Work out the finished part from the listing and answer in its coordinate system (mm). Coordinates: 2 decimals unless noted, no trailing zeros.
1. The part is cut by section A-A, the plane z = -34.6. Count the separate pieces of the cut face and the enclosed holes in it, then the cut area to 3 significant figures.
2. Flat-ended cylindrical pins translate along their axes: pin 1 Ø1 at (x, y) = (-28.5, -25.5) entering from +Z; pin 2 Ø1.5 at (y, z) = (-20.5, -35.5) entering from +X; pin 3 Ø2 at (x, y) = (19.5, -22.5) entering from +Z. Find the tip coordinate at first contact, or state that the pin passes through.
3. Find the intervals of material crossed by probe 1 along X at (y, z) = (-22.75, -34.7); probe 2 along X at (y, z) = (-23, -36.3); probe 3 along Y at (x, z) = (-55.5, -36.2), in increasing order.
```python
from build123d import *

# Parameters (mm, degrees)
BOX126_W                          = 90
BOX126_H                          = 9
BOX126_DEPTH                      = 4
BOX125_W                          = 40
BOX125_H                          = 10
BOX125_DEPTH                      = 10
CYLINDER211_R                     = 3.25
CYLINDER211_DEPTH                 = 3.5
CYLINDER212_R                     = 0.6
CYLINDER212_DEPTH                 = 9.5
CYLINDER210_R                     = 0.6
CYLINDER210_DEPTH                 = 9.5
CYLINDER209_R                     = 3.25
CYLINDER209_DEPTH                 = 3.5
PAD016_DEPTH                      = 4
FILLET087_R                       = 3
PART_MIRRORING004_PLACEMENT_ANGLE = 180
BOX123_W                          = 40
BOX123_H                          = 10
BOX123_DEPTH                      = 10
CYLINDER205_R                     = 3.25
CYLINDER205_DEPTH                 = 3.5
CYLINDER208_R                     = 0.6
CYLINDER208_DEPTH                 = 9.5
CYLINDER206_R                     = 0.6
CYLINDER206_DEPTH                 = 9.5
CYLINDER207_R                     = 3.25
CYLINDER207_DEPTH                 = 3.5
PAD017_DEPTH                      = 4
FILLET086_R                       = 3


with BuildPart() as obj1:
    # Box126 → Box126 (new body)
    with BuildSketch(Plane(origin=(-63, -27.5, -41), x_dir=(1, 0, 0), z_dir=(0, 0, 1))):
        with Locations((45, 4.5)):
            Rectangle(BOX126_W, BOX126_H)
    extrude(amount=BOX126_DEPTH)


with BuildPart() as obj2:
    # Box125 → Box125 (new body)
    with BuildSketch(Plane(origin=(-14, -72, -42), x_dir=(1, 0, 0), z_dir=(0, 0, 1))):
        with Locations((20, 5)):
            Rectangle(BOX125_W, BOX125_H)
    extrude(amount=BOX125_DEPTH)


with BuildPart() as zylinder211:
    # Cylinder211 → Cylinder211 (new body)
    with BuildSketch(Plane(origin=(-52.5, 23, -36), x_dir=(1, 0, 0), z_dir=(0, 0, 1))):
        Circle(CYLINDER211_R)
    extrude(amount=CYLINDER211_DEPTH)


with BuildPart() as zylinder212:
    # Cylinder212 → Cylinder212 (new body)
    with BuildSketch(Plane(origin=(16.5, 23, -39), x_dir=(1, 0, 0), z_dir=(0, 0, 1))):
        Circle(CYLINDER212_R)
    extrude(amount=CYLINDER212_DEPTH)


with BuildPart() as zylinder210:
    # Cylinder210 → Cylinder210 (new body)
    with BuildSketch(Plane(origin=(-52.5, 23, -39), x_dir=(1, 0, 0), z_dir=(0, 0, 1))):
        Circle(CYLINDER210_R)
    extrude(amount=CYLINDER210_DEPTH)


with BuildPart() as fusion135:
    # Cylinder209 → Cylinder209 (new body)
    with BuildSketch(Plane(origin=(16.5, 23, -36), x_dir=(1, 0, 0), z_dir=(0, 0, 1))):
        Circle(CYLINDER209_R)
    extrude(amount=CYLINDER209_DEPTH)

    # Fusion135: union Zylinder211, Zylinder212, Zylinder210
    add(zylinder211.part)
    add(zylinder212.part)
    add(zylinder210.part)


with BuildPart() as cut090:
    # Sketch017 → Pad016 (new body)
    with BuildSketch(Plane.XY):
        with BuildLine():
            add(Edge.make_bspline(
                [(-48.5, 19), (-18, 24), (12.5, 19)],
                knots=[0, 0, 0, 1, 1, 1], degree=2))
            Line((-48.5, 19), (-57, 19))
            Line((-57, 19), (-57, 27))
            Line((-57, 27), (-48.5, 27))
            add(Edge.make_bspline(
                [(-48.5, 27), (-18, 22), (12.5, 27)],
                knots=[0, 0, 0, 1, 1, 1], degree=2))
            Line((12.5, 27), (21, 27))
            Line((21, 27), (21, 19))
            Line((21, 19), (12.5, 19))
        make_face()
    extrude(amount=PAD016_DEPTH)


with BuildPart() as cut090_1:
    # Body007 placement: moved
    add(cut090.part.moved(Location((0, 0, -38))))

    # Cut088: cut Fusion135
    add(fusion135.part, mode=Mode.SUBTRACT)

    # Fillet087
    fillet087_edges = [cut090_1.edges().sort_by_distance(p)[0] for p in [
        (-57, 19, -36),
        (21, 19, -36),
        (-57, 27, -36),
        (21, 27, -36),
    ]]
    fillet(fillet087_edges, radius=FILLET087_R)


with BuildPart() as cut090_2:
    # Fillet087 placement: moved
    add(cut090_1.part.moved(Location((0, -90, 0))))

    # Cut090: cut obj2
    add(obj2.part, mode=Mode.SUBTRACT)


with BuildPart() as cut090_3:
    # Cut090 placement: moved
    add(cut090_2.part.moved(Location((-5, 35, 0))))


with BuildPart() as part_mirroring004:
    # Part__Mirroring004: instance of Cut090
    add(cut090_3.part.mirror(Plane(origin=(-40.5, -8e-06, -36), x_dir=(1, 0, 0), z_dir=(0, 1, 0))))


with BuildPart() as part_mirroring004_1:
    # Part__Mirroring004 placement: moved
    add(part_mirroring004.part.moved(Location((-38, 9, 0))).rotate(Axis((-38, 9, 0), (0, 0, 1)), PART_MIRRORING004_PLACEMENT_ANGLE))


with BuildPart() as obj3:
    # Box123 → Box123 (new body)
    with BuildSketch(Plane(origin=(-14, -72, -42), x_dir=(1, 0, 0), z_dir=(0, 0, 1))):
        with Locations((20, 5)):
            Rectangle(BOX123_W, BOX123_H)
    extrude(amount=BOX123_DEPTH)


with BuildPart() as zylinder205:
    # Cylinder205 → Cylinder205 (new body)
    with BuildSketch(Plane(origin=(-52.5, 23, -36), x_dir=(1, 0, 0), z_dir=(0, 0, 1))):
        Circle(CYLINDER205_R)
    extrude(amount=CYLINDER205_DEPTH)


with BuildPart() as zylinder208:
    # Cylinder208 → Cylinder208 (new body)
    with BuildSketch(Plane(origin=(16.5, 23, -39), x_dir=(1, 0, 0), z_dir=(0, 0, 1))):
        Circle(CYLINDER208_R)
    extrude(amount=CYLINDER208_DEPTH)


with BuildPart() as zylinder206:
    # Cylinder206 → Cylinder206 (new body)
    with BuildSketch(Plane(origin=(-52.5, 23, -39), x_dir=(1, 0, 0), z_dir=(0, 0, 1))):
        Circle(CYLINDER206_R)
    extrude(amount=CYLINDER206_DEPTH)


with BuildPart() as fusion134:
    # Cylinder207 → Cylinder207 (new body)
    with BuildSketch(Plane(origin=(16.5, 23, -36), x_dir=(1, 0, 0), z_dir=(0, 0, 1))):
        Circle(CYLINDER207_R)
    extrude(amount=CYLINDER207_DEPTH)

    # Fusion134: union Zylinder205, Zylinder208, Zylinder206
    add(zylinder205.part)
    add(zylinder208.part)
    add(zylinder206.part)


with BuildPart() as bar_medium_long:
    # Sketch016 → Pad017 (new body)
    with BuildSketch(Plane.XY):
        with BuildLine():
            add(Edge.make_bspline(
                [(-48.5, 19), (-18, 24), (12.5, 19)],
                knots=[0, 0, 0, 1, 1, 1], degree=2))
            Line((-48.5, 19), (-57, 19))
            Line((-57, 19), (-57, 27))
            Line((-57, 27), (-48.5, 27))
            add(Edge.make_bspline(
                [(-48.5, 27), (-18, 22), (12.5, 27)],
                knots=[0, 0, 0, 1, 1, 1], degree=2))
            Line((12.5, 27), (21, 27))
            Line((21, 27), (21, 19))
            Line((21, 19), (12.5, 19))
        make_face()
    extrude(amount=PAD017_DEPTH)


with BuildPart() as bar_medium_long_1:
    # Body008 placement: moved
    add(bar_medium_long.part.moved(Location((0, 0, -38))))

    # Cut086: cut Fusion134
    add(fusion134.part, mode=Mode.SUBTRACT)

    # Fillet086
    fillet086_edges = [bar_medium_long_1.edges().sort_by_distance(p)[0] for p in [
        (-57, 19, -36),
        (21, 19, -36),
        (-57, 27, -36),
        (21, 27, -36),
    ]]
    fillet(fillet086_edges, radius=FILLET086_R)


with BuildPart() as bar_medium_long_2:
    # Fillet086 placement: moved
    add(bar_medium_long_1.part.moved(Location((0, -90, 0))))

    # Cut087: cut obj3
    add(obj3.part, mode=Mode.SUBTRACT)


with BuildPart() as bar_medium_long_3:
    # Cut087 placement: moved
    add(bar_medium_long_2.part.moved(Location((-3, 44, 0))))

    # Fusion136: union Part__Mirroring004
    add(part_mirroring004_1.part)

    # Cut091: cut obj1
    add(obj1.part, mode=Mode.SUBTRACT)


solid = bar_medium_long_3.part
```
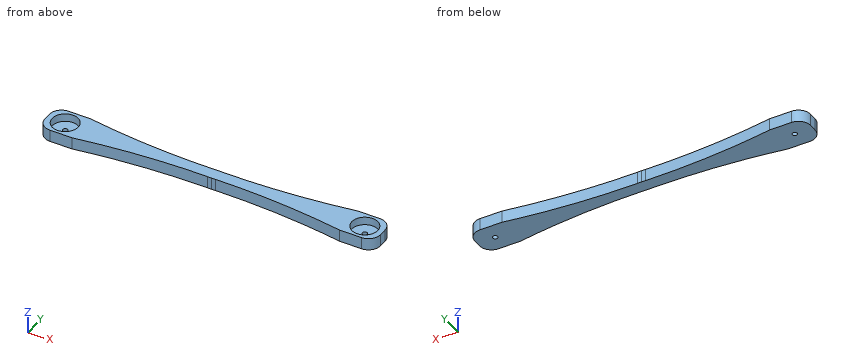
Geometry says:
1. separate pieces: 1
1. enclosed holes: 2
1. area: 365 mm2
2. pin 1: passes through
2. pin 2: stops at x = 23.9
2. pin 3: stops at z = -36
3. probe 1: x = -60 to -58.74, -52.26 to 16.26, 22.74 to 24
3. probe 2: x = -60 to -56.1, -54.9 to 18.9, 20.1 to 24
3. probe 3: y = -27 to -23.6, -22.4 to -19
